Design review of the part built by this model. Coordinates are the model's own, in mm. A direction names the side the tool comes from. Coordinates: 2 decimals unless noted, no trailing zeros. Loops run counter-clockwise (first coordinate to the right, second up) from the corner with the lowest first, then second, coordinate; pieces in that order, holes last. Notation, with made-up numbers: M 44.25,-30 L 94.25,-30 A35 cw 94.25,5 Z; hole C 14.5,-27 d9. An arc over 180 degrees is marked long. Answer as CSV lines item,"result". Start each with the question number.
from build123d import *

# Parameters (mm, degrees)
SKETCH3_W            = 95.25
SKETCH3_H            = 60.96
BOSS_EXTRUDE1_DEPTH  = 6.35
SKETCH4_W            = 6.56336
SKETCH4_H            = 45.72
SKETCH4_W_2          = 9.8836988
CUT_EXTRUDE1_DEPTH   = 6.35
SKETCH5_W            = 5.1689
SKETCH5_H            = 6.7564
CUT_EXTRUDE2_DEPTH   = 57.898976485
SKETCH9_W            = 95.25
SKETCH9_H            = 6.35
CUT_EXTRUDE6_DEPTH   = 8.89
SKETCH11_W           = 82.12328
SKETCH11_H           = 6.35
CUT_EXTRUDE9_DEPTH   = 7.62
M6_CLEARANCE_HOLE2_D = 7


with BuildPart() as part:
    # Sketch3 → Boss-Extrude1 (new body)
    with BuildSketch(Plane.XY):
        Rectangle(SKETCH3_W, SKETCH3_H)
    extrude(amount=BOSS_EXTRUDE1_DEPTH)

    # Sketch4 → Cut-Extrude1 (cut)
    with BuildSketch(Plane.XY.offset(6.35)):
        with Locations((-44.34332, -7.62)):
            Rectangle(SKETCH4_W, SKETCH4_H)
        with Locations((0, -7.62)):
            Rectangle(SKETCH4_W_2, SKETCH4_H)
        with Locations((44.34332, -7.62)):
            Rectangle(SKETCH4_W, SKETCH4_H)
    extrude(amount=-CUT_EXTRUDE1_DEPTH, mode=Mode.SUBTRACT)

    # Sketch5 → Cut-Extrude2 (cut, through all)
    with BuildSketch(Plane.XY.offset(6.35)):
        with Locations((-38.68039, 12.065)):
            Rectangle(SKETCH5_W, SKETCH5_H)
        with Locations((-7.3230994, 12.065)):
            Rectangle(SKETCH5_W, SKETCH5_H)
    cut_extrude2 = extrude(amount=-CUT_EXTRUDE2_DEPTH, mode=Mode.SUBTRACT)

    # Mirror1: Cut-Extrude2 across plane
    add(cut_extrude2.mirror(Plane(origin=(0, 0, 0), x_dir=(0, 0, 1), z_dir=(1, 0, 0))), mode=Mode.SUBTRACT)

    # Sketch9 → Cut-Extrude6 (cut)
    with BuildSketch(Plane(origin=(0, 30.48, 0), x_dir=(1, 0, 0), z_dir=(0, 1, 0))):
        with Locations((0, -3.175)):
            Rectangle(SKETCH9_W, SKETCH9_H)
    extrude(amount=-CUT_EXTRUDE6_DEPTH, mode=Mode.SUBTRACT)

    # Sketch11 → Cut-Extrude9 (cut)
    with BuildSketch(Plane.XZ.offset(30.48)):
        with Locations((0, 3.175)):
            Rectangle(SKETCH11_W, SKETCH11_H)
    extrude(amount=-CUT_EXTRUDE9_DEPTH, mode=Mode.SUBTRACT)

    # M6 Clearance Hole2 (through all)
    with Locations(Plane.XY.offset(6.35)):
        with Locations((26, -10.6279), (-26, -10.6279)):
            Hole(M6_CLEARANCE_HOLE2_D / 2)


solid = part.part
Item 1: Add section A-A (x = -26). Give the boundary of the cut face in (y, z).
Item 2: Add section D-D (z = 2.5). Give the number of separate pieces and of enclosed holes in the cut face, plus the area to 3 significant figures.
Item 3: For pin 1 (1.9 mm diameter, centred on y = -10, z = 3, fed in from -X); pin 2 (3 mm diameter, centred on y = -6.5, z = 2, fed in from +X); pin 3 (4 mm diameter, centred on x = 26, y = -10.63, fed in from +Z), all flat-tipped, find the tip position at first contact; note any pin that passes through.
Item 4: For line 1 along Y through (x, z) = (26, 3.5); line 2 along Y through (x, z) = (-41, 1); line 3 along X through (y, z) = (-5, 2.75), list the stretches that pass through material, from the lowest coordinate up. Write a range as from..to.
Item 5: For faces 1 (the face through (39, 8.687, 3)), 2 (the face through (-9.908, 12, 3)), 3 (the face through (-39, 8.687, 3)), list the 3-axis set-ups (+Z, -Z, +X, -X, +Y, -Y) from which the entire face can be reached by the end or side of a thin tool; tool diameter is ignored.
Item 6: Add section C-C (y = -12). Give the boundary of the cut face in (x, z).
Item 7: Mouldability with a two-part tool opening along Y and no side actions: class faces 4 (the face through (23, -22.86, 3)), 5 (the face through (36.096, 12, 3)), 6 (the face through (-41.062, -7, 3)) as released by +Y, released by -Y, zero draft, split by the parting line, or undercut.
Item 8: Add section B-B (y = -19). Give the boundary of the cut face in (x, z), plus the area to 3 significant figures.
Response:
1,outline,"M -22.86,0 L -14.13,0 L -14.13,6.35 L -22.86,6.35 Z; M -7.13,0 L 21.59,0 L 21.59,6.35 L -7.13,6.35 Z"
2,separate pieces,"1"
2,enclosed holes,"2"
2,area,"3,150 mm²"
3,pin 1,"x = -41.06"
3,pin 2,"x = 41.06"
3,pin 3,"through"
4,line 1,"-22.86..-14.13, -7.13..21.59"
4,line 2,"-22.86..8.69, 15.44..21.59"
4,line 3,"-41.06..-4.94, 4.94..41.06"
5,face 1,"+Z, -Z, +X"
5,face 2,"+Z, -Z"
5,face 3,"+Z, -Z, -X"
6,outline,"M -41.06,0 L -29.22,0 L -29.22,6.35 L -41.06,6.35 Z; M -22.78,0 L -4.94,0 L -4.94,6.35 L -22.78,6.35 Z; M 4.94,0 L 22.78,0 L 22.78,6.35 L 4.94,6.35 Z; M 29.22,0 L 41.06,0 L 41.06,6.35 L 29.22,6.35 Z"
7,face 4,"released by -Y"
7,face 5,"undercut"
7,face 6,"zero draft"
8,outline,"M -41.06,0 L -4.94,0 L -4.94,6.35 L -41.06,6.35 Z; M 4.94,0 L 41.06,0 L 41.06,6.35 L 4.94,6.35 Z"
8,area,"459 mm²"
